Geometry check sheet. Reference: the model listing, model coordinates, mm. A direction names the side the tool comes from. Coordinates: 2 decimals unless noted, no trailing zeros. Order: outer loops, then holes, each group sorted by start corner. A loop starts at its lowest first (then second) coordinate and runs counter-clockwise, first axis right, second up. Notation, with made-up numbers: M 50.25,62 L 103.25,62 A19 cw 103.25,69 Z; hole C 43,-3.5 d4. An arc over 180 degrees is marked long. Use CSV: the item, a comma, the result in double quotes. Start each with the question number.
```python
from build123d import *

# Parameters (mm, degrees)
ESQUISSE1_R             = 15
BOSS_EXTRU_1_DEPTH      = 45
ESQUISSE4_R             = 9.5
ENL_V_MAT_EXTRU_3_DEPTH = 7
ENL_V_START             = -7
ESQUISSE5_R             = 9.5
ENL_V_MAT_EXTRU_4_DEPTH = 7
ESQUISSE6_R             = 8
ENL_V_MAT_EXTRU_5_DEPTH = 60
CONG_1_R                = 3


with BuildPart() as part:
    # Esquisse1 → Boss.-Extru.1 (new body)
    with BuildSketch(Plane.XY):
        with Locations(Location((0, 0, 0), (0, 0, 180))):
            Circle(ESQUISSE1_R)
    extrude(amount=BOSS_EXTRU_1_DEPTH)

    # Esquisse4 → Enlèv. mat.-Extru.3 (cut)
    with BuildSketch(Plane.XY.offset(45)):
        Circle(ESQUISSE4_R)
    extrude(amount=-ENL_V_MAT_EXTRU_3_DEPTH, mode=Mode.SUBTRACT)

    # Esquisse5 → Enlèv. mat.-Extru.4 (cut)
    with BuildSketch(Plane(origin=(0, 0, 0), x_dir=(-1, 0, 0), z_dir=(0, 0, -1)).offset(ENL_V_START)):
        with Locations(Location((0, 0, 0), (0, 0, 180))):
            Circle(ESQUISSE5_R)
    extrude(amount=ENL_V_MAT_EXTRU_4_DEPTH, mode=Mode.SUBTRACT)

    # Esquisse6 → Enlèv. mat.-Extru.5 (cut)
    with BuildSketch(Plane(origin=(0, 0, 7), x_dir=(-1, 0, 0), z_dir=(0, 0, -1))):
        Circle(ESQUISSE6_R)
    extrude(amount=-ENL_V_MAT_EXTRU_5_DEPTH, mode=Mode.SUBTRACT)

    # Congé1
    cong_1_edges = [part.edges().sort_by_distance(p)[0] for p in [
        (15, 0, 0),
        (15, 0, 45),
    ]]
    fillet(cong_1_edges, radius=CONG_1_R)


solid = part.part
```
1) Gauge pin test, flat ends, axial feed: P1, Ø9.5, axis at x = -3.5, y = 2, coming from the +Z side; P2, Ø2, axis at y = -4.5, z = 22, coming from the +X side; P3, Ø1, axis at x = 6, z = 23, coming from the -Y side; P4, Ø5.5, axis at x = -1, y = 2.5, coming from the -Z side. Record the tip position at first contact, or that the pin passes through.
2) Draft check along Y on faces 1 (the face through (-8.06, -12.65, 22.23)), 2 (the face through (-9, -4, 45)), 3 (the face through (1.73, -7.81, 22.28)). Enter one of: +Y half, -Y half, draft (parallel to the pull), parting line (faces both ways), or undercut.
3) Section check C-C on z = 39.5. Record the boundary of the cut face in (x, y).
4) Section check A-A on y = 0. Record the boundary of the cut face in (x, z), then the cut area to 3 significant figures.
5) Material ranges on line 1 along Y through (x, z) = (0, 14.5); line 2 along Y through (x, z) = (0, 41.25); line 3 along X through (y, z) = (-9, 35), recorded low to high.
6) Set-up check for faces 4 (the face through (-4.3, 7, 7)), 5 (the face through (-9, -4, 0)), 6 (the face through (4.38, -8.43, 41.55)): record each of +Z, -Z, +X, -X, +Y, -Y from which the full face is reachable in a straight line by a thin tool's end or side.
7) Section check D-D on z = 22.5. Record the boundary of the cut face in (x, y).
Results are:
1,P1,"stops at z = 38"
1,P2,"stops at x = 14.59"
1,P3,"stops at y = -13.96"
1,P4,"passes through"
2,face 1,"parting line"
2,face 2,"draft"
2,face 3,"undercut"
3,outline,"C 0,0 d30; hole C 0,0 d19"
4,outline,"M -15,3 A3 ccw -12,0 L -9.5,0 L -9.5,7 L -8,7 L -8,38 L -9.5,38 L -9.5,45 L -12,45 A3 ccw -15,42 Z; M 8,7 L 9.5,7 L 9.5,0 L 12,0 A3 ccw 15,3 L 15,42 A3 ccw 12,45 L 9.5,45 L 9.5,38 L 8,38 Z"
4,area,"580 mm²"
5,line 1,"y = -15 to -8, 8 to 15"
5,line 2,"y = -15 to -9.5, 9.5 to 15"
5,line 3,"x = -12 to 12"
6,face 4,"-Z"
6,face 5,"-Z, +X, -X, +Y, -Y"
6,face 6,"+Z"
7,outline,"C 0,0 d30; hole C 0,0 d16"
